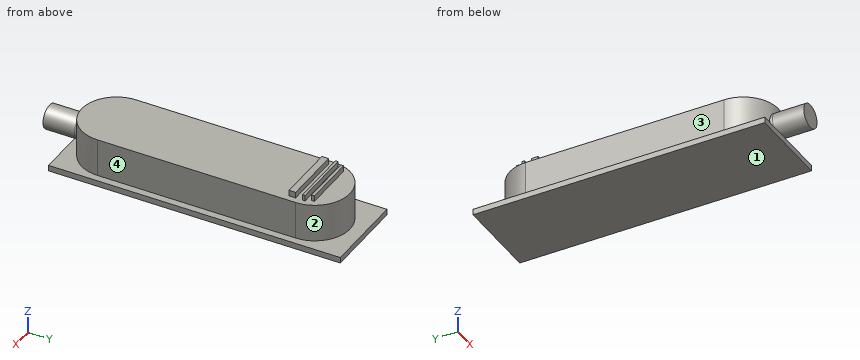
```python
from build123d import *

# Parameters (mm, degrees)
SKETCH1_W           = 14.477015864
SKETCH1_H           = 50.012098532
BOSS_EXTRUDE1_DEPTH = 1
BOSS_EXTRUDE2_DEPTH = 6.5
SKETCH4_W           = 9.051394426
SKETCH4_H           = 0.494998133
SKETCH4_W_2         = 10.182818728
SKETCH4_H_2         = 0.424284113
SKETCH4_H_3         = 1.131424304
BOSS_EXTRUDE4_DEPTH = 1
SCALE1_SCALE        = 0.5
SCALE2_SCALE        = 0.5
SKETCH5_R           = 0.511212816
BOSS_EXTRUDE5_DEPTH = 1.35
SKETCH7_R           = 0.511212816
BOSS_EXTRUDE6_DEPTH = 1.35


with BuildPart() as part:
    # Sketch1 → Boss-Extrude1 (new body)
    with BuildSketch(Plane.XY):
        Rectangle(SKETCH1_W, SKETCH1_H)
    extrude(amount=BOSS_EXTRUDE1_DEPTH)

    # Sketch2 → Boss-Extrude2 (add)
    with BuildSketch(Plane.XY.offset(1)):
        with BuildLine():
            Line((6, 16.665360906), (6, -17.334639094))
            ThreePointArc((6, -17.334639094), (0, -23.334639094), (-6, -17.334639094))
            Line((-6, -17.334639094), (-6, 16.665360906))
            ThreePointArc((-6, 16.665360906), (0, 22.665360906), (6, 16.665360906))
        make_face()
    extrude(amount=BOSS_EXTRUDE2_DEPTH)

    # Sketch4 → Boss-Extrude4 (add)
    with BuildSketch(Plane.XY.offset(7.5)):
        with Locations((-0.141428038, 18.743662091)):
            Rectangle(SKETCH4_W, SKETCH4_H)
        with Locations((-0.141428038, 17.506166759)):
            Rectangle(SKETCH4_W_2, SKETCH4_H_2)
        with Locations((-0.141428038, 15.526174228)):
            Rectangle(SKETCH4_W_2, SKETCH4_H_3)
    extrude(amount=BOSS_EXTRUDE4_DEPTH)


with BuildPart() as part_1:
    # Scale1: scaled about (-0.000695656, -0.192418976, 3.611272537)
    add(part.part.scale(SCALE1_SCALE).moved(Location((-0.000347828, -0.096209488, 1.805636269))))


with BuildPart() as part_2:
    # Scale2: scaled about (-0.000695656, -0.192418976, 3.611272537)
    add(part_1.part.scale(SCALE2_SCALE).moved(Location((-0.000347828, -0.096209488, 1.805636269))))



with BuildPart() as body_2:
    # Sketch5 → Boss-Extrude5 (new body)
    with BuildSketch(Plane(origin=(0, -6, 0), x_dir=(1, 0, 0), z_dir=(0, 1, 0))):
        with Locations(Location((0, -3.78422441, 0), (0, 0, 270))):
            Circle(SKETCH5_R)
    extrude(amount=-BOSS_EXTRUDE5_DEPTH)


with BuildPart() as part_3:
    add(part_2.part)

    add(body_2.part)  # Boss-Extrude6 merges body 2
    # Sketch7 → Boss-Extrude6 (add)
    with BuildSketch(Plane(origin=(0, -6, 0), x_dir=(1, 0, 0), z_dir=(0, 1, 0))):
        with Locations(Location((0, -3.78422441, 0), (0, 0, 90))):
            Circle(SKETCH7_R)
    extrude(amount=BOSS_EXTRUDE6_DEPTH)


solid = part_3.part
```
For this review, take the finished solid that the model builds, in its own axes (mm). Face numbers are marked on the shaded views. A direction names the side the tool comes from. Give positions to 0.01 mm unless a question says otherwise; leave off trailing zeros. Order: outer loops, then holes, each group sorted by start corner. A loop starts at its lowest first (then second) coordinate and runs counter-clockwise, first axis right, second up.
1) Take a section at A-A (y = -6.25). Give the boundary of the cut face in (x, z), then the cut area to 3 significant figures.
2) Take a section at D-D (z = 3.85). Give the boundary of the cut face in (x, y), then the cut area to 3 significant figures.
3) Wall thickness on line 1 (X direction, y = 3.75, z = 3.95); line 2 (Z direction, x = -0.9, y = 1); line 3 (Y direction, x = 0.1, z = 3.9): over which ranges is each line inside the solid? List them lowest first.
4) Take a section at B-B (x = 0). Give the boundary of the cut face in (y, z), then the cut area to 3 significant figures.
5) Insertion check: pin 1 (2 mm diameter, centred on x = 0.5, y = 0, fed in from +Z); pin 2 (0.8 mm diameter, centred on y = -1.5, z = 4, fed in from -X). Each pin has a flat end and moves straight along its axis. Give the tip position at first contact, or say it passes through.
6) Take a section at C-C (y = -1). Give the boundary of the cut face in (x, z).
7) For the marked faces 1, 2, 3 and 4, list the 3-axis set-ups (+Z, -Z, +X, -X, +Y, -Y) from which the entire face can be reached by the end or side of a thin tool; tool diameter is ignored.
Derived:
1. outline: (-1.81, 2.71) - (1.81, 2.71) - (1.81, 2.96) - (-1.81, 2.96) - close; circle Ø1.02 at (0, 3.78)
1. area: 1.73 mm2
2. outline: (-1.5, -4.48) arc R1.5 ccw to (-0.51, -5.89) - (-0.51, -7.35) - (0.51, -7.35) - (0.51, -5.89) arc R1.5 ccw to (1.5, -4.48) - (1.5, 4.02) arc R1.5 ccw to (-1.5, 4.02) - close
2. area: 34.0 mm2
3. line 1: x = -1.5 to 1.5
3. line 2: z = 2.71 to 4.58
3. line 3: y = -7.35 to 5.52
4. outline: (-7.35, 3.27) - (-5.98, 3.27) - (-5.98, 2.96) - (-6.4, 2.96) - (-6.4, 2.71) - (6.11, 2.71) - (6.11, 2.96) - (5.52, 2.96) - (5.52, 4.58) - (4.6, 4.58) - (4.6, 4.83) - (4.48, 4.83) - (4.48, 4.58) - (4.29, 4.58) - (4.29, 4.83) - (4.18, 4.83) - (4.18, 4.58) - (3.88, 4.58) - (3.88, 4.83) - (3.6, 4.83) - (3.6, 4.58) - (-5.98, 4.58) - (-5.98, 4.3) - (-7.35, 4.3) - close
4. area: 23.3 mm2
5. pin 1: stops at z = 4.58
5. pin 2: stops at x = -1.5
6. outline: (-1.81, 2.71) - (1.81, 2.71) - (1.81, 2.96) - (1.5, 2.96) - (1.5, 4.58) - (-1.5, 4.58) - (-1.5, 2.96) - (-1.81, 2.96) - close
7. face 1: -Z, +X, -X, +Y, -Y
7. face 2: +Z, +Y
7. face 3: +Z, -X, +Y, -Y
7. face 4: +Z, +X, +Y, -Y
